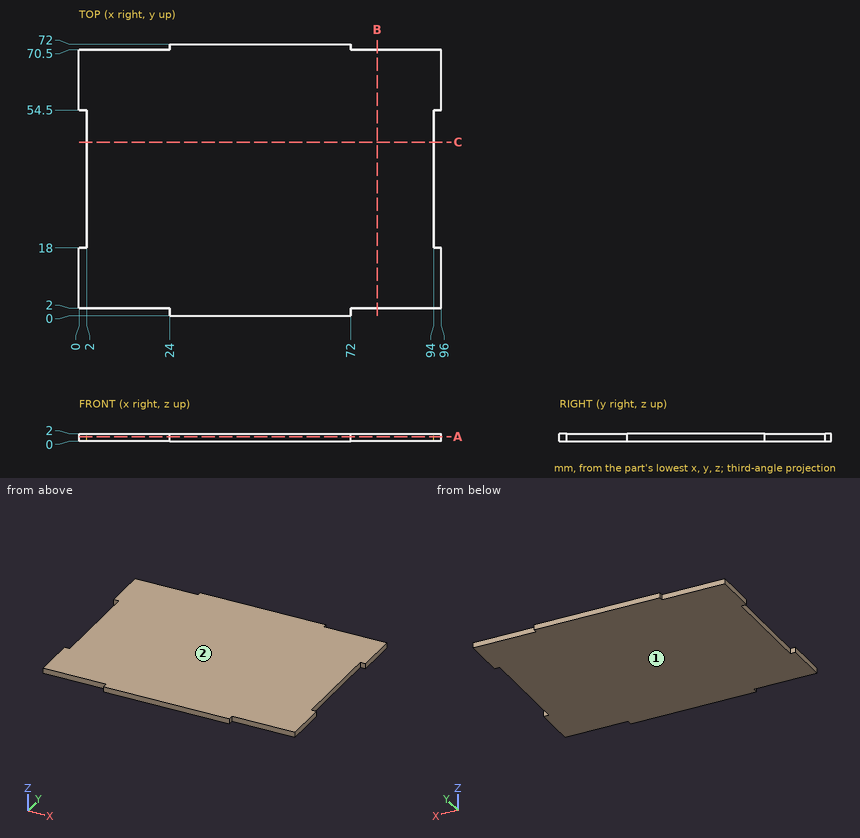
Verification items for this drawing (mm, ordinates from the low corner). Coordinates: 2 decimals unless noted, no trailing zeros. Loops run counter-clockwise (first coordinate to the right, second up) from the corner with the lowest first, then second, coordinate; pieces in that order, holes last. Notation, with made-up numbers: (58, -27.75) - (94, -27.75) arc R20 cw to (94, -11.75) - close; hole circle Ø5 at (-35, 26). An arc over 180 degrees is marked (long way). Use one line per item in the form item = value. Start each with the question number.
Item 1: Section check A-A, the plane z = 1.25. Enter the section's corners in (x, y), and give its area (3 significant figures).
Item 2: Section check B-B, the plane x = 79. Enter the section's corners in (y, z), and give its area (3 significant figures).
Item 3: Thickness scan on probe 1 along Y at (x, z) = (8, 1); probe 2 along X at (y, z) = (46, 1.15). Record the ranges inside material, lowest first.
Item 4: Section check C-C, the plane y = 46. Enter the section's corners in (x, z), and give its area (3 significant figures).
Item 5: Gauge pin test, flat ends, axial feed: pin 1 (0.6 mm diameter, centred on y = 1.5, z = 0.5, fed in from -X); pin 2 (0.6 mm diameter, centred on y = 36.5, z = 1.5, fed in from -X); pin 3 (1 mm diameter, centred on x = 79, z = 1, fed in from -Y); pin 4 (1.5 mm diameter, centred on x = 85, y = 58.5, fed in from -Z). Record the tip position at first contact, or that the pin passes through.
Item 6: Mould release check, pull along Z, two halves, no side actions. Record for the marked faces 1 and 2: +Z half, -Z half, draft (parallel to the pull), parting line (faces both ways), or undercut.
Computed:
q1.outline = (0, 2) - (24, 2) - (24, 0) - (72, 0) - (72, 2) - (96, 2) - (96, 18) - (94, 18) - (94, 54.5) - (96, 54.5) - (96, 70.5) - (72, 70.5) - (72, 72) - (24, 72) - (24, 70.5) - (0, 70.5) - (0, 54.5) - (2, 54.5) - (2, 18) - (0, 18) - close
q1.area = 6,600 mm2
q2.outline = (2, 0) - (70.5, 0) - (70.5, 2) - (2, 2) - close
q2.area = 137 mm2
q3.probe_1 = 2 to 70.5
q3.probe_2 = 2 to 94
q4.outline = (2, 0) - (94, 0) - (94, 2) - (2, 2) - close
q4.area = 184 mm2
q5.pin_1 = 24
q5.pin_2 = 2
q5.pin_3 = 2
q5.pin_4 = 0
q6.face_1 = -Z half
q6.face_2 = +Z half
